```python
from build123d import *

# Parameters (mm, degrees)
F1_DEPTH = 50
F2_R     = 2
F2_R_2   = 4
F3_DEPTH = 8
F4_R     = 1
F5_DEPTH = 5
F6_R     = 1
F7_DEPTH = 8
F8_R     = 2.5
F8_R_2   = 1
F8_R_3   = 2.689756
F9_DEPTH = 4


with BuildPart() as f1:
    # F0 (on Right) → F1 (new body)
    with BuildSketch(Plane.YZ):
        Polygon((-8.773239, 0), (41.226761, 0), (41.226761, 8), (8, 8), (8, 48), (0, 48), (0, 8), (-8.773239, 8), align=None)
    extrude(amount=F1_DEPTH)

    # F2 (on face) → F3 (cut, through all)
    with BuildSketch(Plane.XZ):
        with Locations((6, 42)):
            Circle(F2_R)
        with Locations((6, 14)):
            Circle(F2_R)
        with Locations((20, 28)):
            Circle(F2_R_2)
        with Locations((34, 42)):
            Circle(F2_R)
        with Locations((34, 14)):
            Circle(F2_R)
    extrude(amount=-F3_DEPTH, mode=Mode.SUBTRACT)

    # F4 (on face) → F5 (cut)
    with BuildSketch(Plane(origin=(0, 0, 0), x_dir=(1, 0, 0), z_dir=(0, 0, -1))):
        with Locations((16, 5.773239)):
            Circle(F4_R)
        with Locations((34, 5.773239)):
            Circle(F4_R)
        with Locations((34, -4.226761)):
            Circle(F4_R)
        with Locations((16, -4.226761)):
            Circle(F4_R)
    extrude(amount=-F5_DEPTH, mode=Mode.SUBTRACT)

    # F6 (on face) → F7 (cut, through all)
    with BuildSketch(Plane.XY.offset(8)):
        with Locations((10, 15)):
            Circle(F6_R)
        with Locations((40, 15)):
            Circle(F6_R)
    extrude(amount=-F7_DEPTH, mode=Mode.SUBTRACT)

    # F8 (on face) → F9 (cut)
    with BuildSketch(Plane.XY.offset(8)):
        with Locations((10, 15)):
            Circle(F8_R)
        with Locations((10, 15)):
            Circle(F8_R_2, mode=Mode.SUBTRACT)
        with Locations((40, 15)):
            Circle(F8_R_3)
        with Locations((40, 15)):
            Circle(F8_R_2, mode=Mode.SUBTRACT)
    extrude(amount=-F9_DEPTH, mode=Mode.SUBTRACT)


solid = f1.part
```
Could you check a few things on this model? Use its own coordinates, in mm. A direction names the side the tool comes from. Round coordinates to 2 decimals unless told otherwise and drop trailing zeros. Write each loop counter-clockwise with the first axis right and the second up, starting at its lowest first coordinate (ties: lowest second). Pieces come first, ordered by that corner, then holes. Notation, with made-up numbers: M 59.5,43.25 L 82.5,43.25 A24 cw 82.5,54.25 Z; hole C -7.75,50.25 d2. An arc over 180 degrees is marked long. Answer in a Markdown table with one row per item. Add a question column.
Q1. Imagine slicing it at D-D (x = 34). Please give me the cut outline in (y, z).
Q2. Imagine slicing it at B-B (y = 15). Please give me the cut outline in (x, z).
Q3. Imagine slicing it at C-C (x = 10). Please give me the cut outline in (y, z), then the cut area to 3 significant figures.
Q4. On a 3-axis mill with a long thin cutter (end or side, diameter ignored), from which of +Z, -Z, +X, -X, +Y, -Y can I reach the whole of each face in a straight line? I mean faces 4 (the cylindrical face through (6, 4, 16)), 5 (the flat face through (25, 41.227, 4)), 6 (the flat face through (25, 25, 8)), 7 (the flat face through (11, 14, 4)), 8 (the cylindrical face through (33.783, -4.797, 2.465)). Say none if no direction works.
Q5. If I drill on line 1 (Y direction, x = 16, z = 2); line 2 (Z direction, x = 6, y = 3); line 3 (Y direction, x = 10, z = 2), over which ranges is the centre line in solid material (lowest first)? Write a range as from..to.
Q6. If we mould it in two halves opening along X, with no side actions, what happens to faces 1 (the flat face through (25, -4, 8)), 2 (the flat face through (40, 13.8, 4)), 3 (the flat face through (0, 7, 15))? For each: +X half, -X half, draft (parallel to the pull), parting line (faces both ways), or undercut.
Q7. Will these pins go through, and if not, where does the flat tip stop? pin 1 Ø1.6 at (x, y) = (16, 4.5) entering from -Z; pin 2 Ø1 at (x, z) = (40, 28) entering from +Y; pin 3 Ø2.5 at (x, y) = (31, -4.5) entering from +Z; pin 4 Ø2.5 at (x, z) = (34, 42) entering from -Y.
Q8. Imagine slicing it at A-A (z = 28). Please give me the cut outline in (x, y), then the cut area to 3 significant figures.
Values:
| question | item | result |
|---|---|---|
| 1 | outline | M -8.77,0 L -6.77,0 L -6.77,5 L -4.77,5 L -4.77,0 L 3.23,0 L 3.23,5 L 5.23,5 L 5.23,0 L 41.23,0 L 41.23,8 L 8,8 L 8,12 L 0,12 L 0,8 L -8.77,8 Z; M 0,16 L 8,16 L 8,40 L 0,40 Z; M 0,44 L 8,44 L 8,48 L 0,48 Z |
| 2 | outline | M 0,0 L 9,0 L 9,4 L 7.5,4 L 7.5,8 L 0,8 Z; M 11,0 L 39,0 L 39,4 L 37.31,4 L 37.31,8 L 12.5,8 L 12.5,4 L 11,4 Z; M 41,0 L 50,0 L 50,8 L 42.69,8 L 42.69,4 L 41,4 Z |
| 3 | outline | M -8.77,0 L 14,0 L 14,4 L 12.5,4 L 12.5,8 L 8,8 L 8,48 L 0,48 L 0,8 L -8.77,8 Z; M 16,0 L 41.23,0 L 41.23,8 L 17.5,8 L 17.5,4 L 16,4 Z |
| 3 | area | 692 mm^2 |
| 4 | face 4 | +Y, -Y |
| 4 | face 5 | +Z, -Z, +X, -X, +Y |
| 4 | face 6 | +Z, +X, -X, +Y |
| 4 | face 7 | +Z |
| 4 | face 8 | -Z |
| 5 | line 1 | -8.77..-6.77, -4.77..3.23, 5.23..41.23 |
| 5 | line 2 | 0..12, 16..40, 44..48 |
| 5 | line 3 | -8.77..14, 16..41.23 |
| 6 | face 1 | draft |
| 6 | face 2 | undercut |
| 6 | face 3 | -X half |
| 7 | pin 1 | z = 0 |
| 7 | pin 2 | y = 8 |
| 7 | pin 3 | z = 8 |
| 7 | pin 4 | through |
| 8 | outline | M 0,0 L 16,0 L 16,8 L 0,8 Z; M 24,0 L 50,0 L 50,8 L 24,8 Z |
| 8 | area | 336 mm^2 |
